Autodesk Inventor part; units mm, degrees
ref_plane "YZ Plane" through (0, 0, 0) normal (1, 0, 0) x (0, 1, 0)
ref_plane "XZ Plane" through (0, 0, 0) normal (0, 1, 0) x (-1, 0, 0)
ref_plane "XY Plane" through (0, 0, 0) normal (0, 0, 1) x (1, 0, 0)
sketch "Sketch1" plane through (0, 0, 0) normal (0, 0, 1) x (1, 0, 0)
  line L0 (0, 0) -> (6, 0)
  line L1 (6, 0) -> (6, 11)
  line L2 (0, 0) -> (0, 15)
  line L3 (0, 15) -> (2, 15)
  line L4 (2, 15) -> (6, 11)
  dimension "d0" = 6
  dimension "d1" = 11
  dimension "d2" = 15
  dimension "d3" = 2
extrude "Extrusion1" add sketch "Sketch1" along normal blind 96
sketch "Sketch2" plane through (0, 0, 0) normal (0, -1, 0) x (1, 0, 0)
  line L0 (0, 0) -> (0, 96)
  line L1 (5.9866, 0) -> (0, 0)
  line L2 (0, 96) -> (6, 96)
  line L3 (0, 96) -> (6, 96)
  line L4 (6, 96) -> (6, 90)
  line L5 (6, 90) -> (0, 96)
  line L6 (0, 0) -> (6, 0)
  line L7 (6, 0) -> (0, 0)
  line L8 (6, 0) -> (6, 6)
  line L9 (6, 0) -> (6, 96)
  line L10 (6, 6) -> (0, 0)
  dimension "d7" = 6
  dimension "d8" = 6
extrude "Extrusion2" cut sketch "Sketch2" against normal blind 42.1125 contours L10 L8 L6 L1 | L2 L4 L5
sketch "Sketch3" plane through (6, 0, 90) normal (1, 0, 0) x (0, 0, -1)
  line L0 (84, 11) -> (0, 11)
  line L1 (84, 0) -> (0, 0)
  line L2 (42, 11) -> (42, 0)
  line L3 (42, 0) -> (48, 0)
  line L4 (90, 0) -> (-6, 0)
  line L5 (48, 0) -> (48, 11)
  line L6 (42, 0) -> (36, 0)
  line L7 (36, 0) -> (36, 11)
  line L8 (42, 11) -> (42, 15)
  line L9 (88, 15) -> (-4, 15)
  line L10 (42, 15) -> (44, 15)
  line L11 (44, 15) -> (48, 11)
  line L12 (42, 15) -> (40, 15)
  line L13 (40, 15) -> (36, 11)
  point P0 (36, 0)
  dimension "d11" = 6
  dimension "d12" = 6
  dimension "d13" = 2
  dimension "d14" = 2
extrude "Extrusion3" add sketch "Sketch3" against normal blind 6
properties part number "edge-join-no-hole"
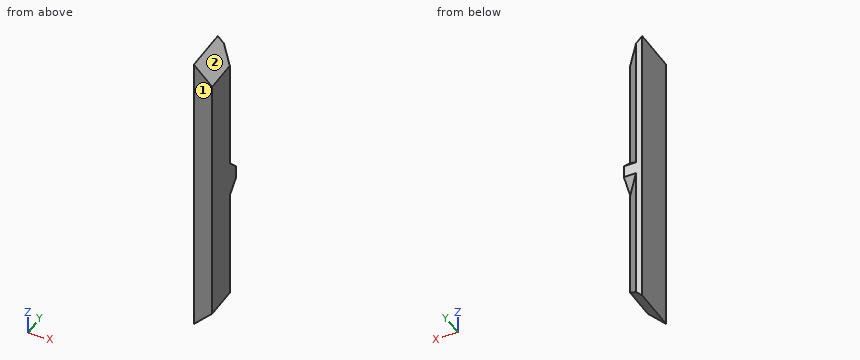
Could you check a few things on this model? Use its own coordinates, in mm. Face numbers are marked on the shaded views. Round coordinates to 2 decimals unless told otherwise and drop trailing zeros. Order: outer loops, then holes, each group sorted by start corner. A loop starts at its lowest first (then second) coordinate and runs counter-clockwise, first axis right, second up. Notation, with made-up numbers: (-25, 73) -> (-6, 73) arc R5 cw to (-6, 81) -> close; hole circle Ø9 at (38, -18.5). An arc over 180 degrees is marked (long way). One line per question, with ' | ' between items.
Q1. I'm going to push a flat-ended pin straight in: pin 1 (3 mm diameter, centred on x = 1, y = 10.5, fed in from +Z). Where does the tip first touch, or does it pass through?
Computed values:
pin 1: z = 96
Q2. If we section it at C-C on z = 38: Write out the boundary of the cut face in (x, y).
Computed values:
outline: (0, 0) -> (6, 0) -> (6, 11) -> (2, 15) -> (0, 15) -> close
Q3. If I drill on line 1 (Z direction, x = 2.25, y = 9.5); line 2 (Z direction, x = 3, y = 0.5); line 3 (Y direction, x = 5, z = 42.5), over which ranges is the centre line in solid material (lowest first)? Write a range as from..to.
Computed values:
line 1: 2.25..93.75 | line 2: 3..93 | line 3: 0..12
Q4. If we section it at B-B on y = 12: Write out the boundary of the cut face in (x, z).
Computed values:
outline: (0, 0) -> (5, 5) -> (5, 43) -> (6, 43) -> (6, 53) -> (5, 53) -> (5, 91) -> (0, 96) -> close
Q5. We'd pull the mould along Y, two halves only. Please class the marked faces 1 and 2: released by +Y, released by -Y, zero draft, split by the parting line, or undercut.
Computed values:
face 1: released by -Y | face 2: zero draft
Q6. If we section it at D-D on y = 1.75: Write out the boundary of the cut face in (x, z).
Computed values:
outline: (0, 0) -> (6, 6) -> (6, 90) -> (0, 96) -> close
Q7. If we section it at A-A on x = 4.5: Write out the boundary of the cut face in (y, z), plus the area to 3 significant figures.
Computed values:
outline: (0, 4.5) -> (12.5, 4.5) -> (12.5, 43.5) -> (15, 46) -> (15, 50) -> (12.5, 52.5) -> (12.5, 91.5) -> (0, 91.5) -> close | area: 1,100 mm²
